Verification items for this drawing (mm, ordinates from the low corner). Give positions to 0.01 mm unless a question says otherwise; leave off trailing zeros. Order: outer loops, then holes, each group sorted by start corner. A loop starts at its lowest first (then second) coordinate and runs counter-clockwise, first axis right, second up. Notation, with made-up numbers: M 73.25,18.5 L 125.25,18.5 A22 cw 125.25,27.5 Z; hole C 47.5,59.25 d11. An arc over 180 degrees is marked long. One line per question, with ' | ' between items. Start each with the question number.
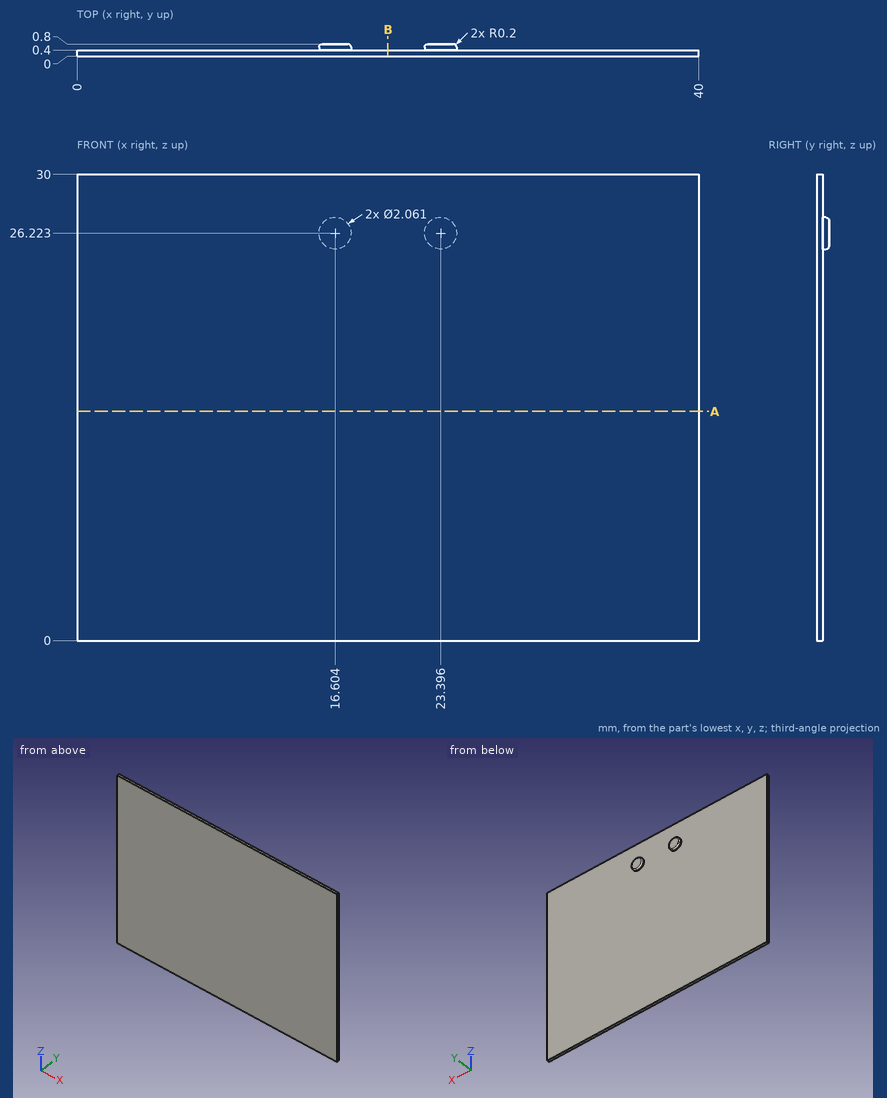
Item 1: Material ranges on line 1 along Y through (x, z) = (24.5, 9.5), recorded low to high.
Item 2: Cross-section at B-B, the plane x = 20. Record the cut outline in (y, z), plus the area to 3 significant figures.
Item 3: Cross-section at A-A, the plane z = 14.75. Record the cut outline in (x, y).
Item 4: Depth check by flat-ended pin: pin 1 (1 mm diameter, centred on x = 7, z = 13, fed in from +Y). Enter the tip coordinate at first touch or a pass-through.
Outcome:
1) line 1: y = 0 to 0.4
2) outline: M 0,0 L 0.4,0 L 0.4,30 L 0,30 Z | area: 12.0 mm²
3) outline: M 0,0 L 40,0 L 40,0.4 L 0,0.4 Z
4) pin 1: stops at y = 0.4
